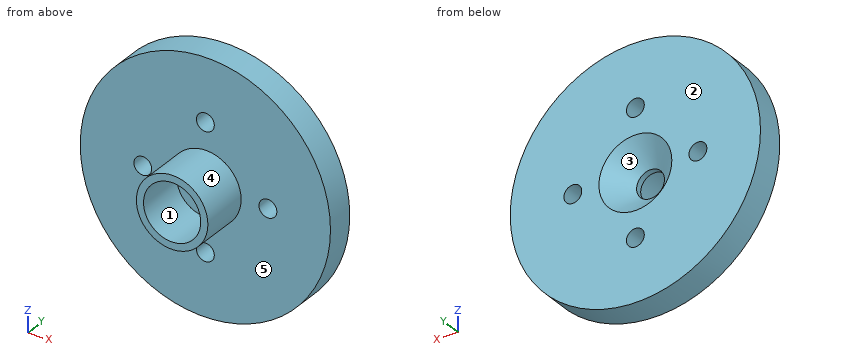
```python
from build123d import *

# Parameters (mm, degrees)
SKETCH1_R                                         = 17.5
BOSS_EXTRUDE1_DEPTH                               = 4
SKETCH2_R                                         = 5
SKETCH2_R_2                                       = 4
BOSS_EXTRUDE2_DEPTH                               = 6.9
SKETCH3_R                                         = 1.25
CUT_EXTRUDE1_DEPTH                                = 6.9
CSK_FOR_M3_5_FLAT_HEAD_MACHINE_SCREW1_D           = 3.9
CSK_FOR_M3_5_FLAT_HEAD_MACHINE_SCREW1_CSINK_D     = 10.2
CSK_FOR_M3_5_FLAT_HEAD_MACHINE_SCREW1_CSINK_ANGLE = 90
SKETCH6_R                                         = 1.25
CUT_EXTRUDE2_DEPTH                                = 6.9


with BuildPart() as part:
    # Sketch1 → Boss-Extrude1 (new body)
    with BuildSketch(Plane(origin=(0, 0, 0), x_dir=(1, 0, 0), z_dir=(0, 1, 0))):
        Circle(SKETCH1_R)
    extrude(amount=BOSS_EXTRUDE1_DEPTH)

    # Sketch2 → Boss-Extrude2 (add)
    with BuildSketch(Plane.XZ):
        Circle(SKETCH2_R)
        Circle(SKETCH2_R_2, mode=Mode.SUBTRACT)
    extrude(amount=BOSS_EXTRUDE2_DEPTH)

    # Sketch3 → Cut-Extrude1 (cut)
    with BuildSketch(Plane.XZ):
        with Locations((-8.75, 0)):
            Circle(SKETCH3_R)
        with Locations((8.75, 0)):
            Circle(SKETCH3_R)
    extrude(amount=-CUT_EXTRUDE1_DEPTH, mode=Mode.SUBTRACT)

    # CSK for M3.5 Flat Head Machine Screw1 (through all)
    with Locations(Plane(origin=(0, 4, 0), x_dir=(1, 0, 0), z_dir=(0, 1, 0))):
        with Locations((0, 0)):
            CounterSinkHole(CSK_FOR_M3_5_FLAT_HEAD_MACHINE_SCREW1_D / 2, CSK_FOR_M3_5_FLAT_HEAD_MACHINE_SCREW1_CSINK_D / 2, counter_sink_angle=CSK_FOR_M3_5_FLAT_HEAD_MACHINE_SCREW1_CSINK_ANGLE)

    # Sketch6 → Cut-Extrude2 (cut)
    with BuildSketch(Plane.XZ):
        with Locations((0, 8.75)):
            Circle(SKETCH6_R)
        with Locations((0, -8.75)):
            Circle(SKETCH6_R)
    extrude(amount=-CUT_EXTRUDE2_DEPTH, mode=Mode.SUBTRACT)


solid = part.part
```
CAD build for the part. Positions are in the model's coordinates, mm. Face numbers are marked on the shaded views. A direction names the side the tool comes from. Round coordinates to 2 decimals unless told otherwise and drop trailing zeros. Order: outer loops, then holes, each group sorted by start corner. A loop starts at its lowest first (then second) coordinate and runs counter-clockwise, first axis right, second up. Notation, with made-up numbers: (40, -31) - (48, -31) arc R6 cw to (48, -26) - close; hole circle Ø5 at (-40, 24.25). An arc over 180 degrees is marked (long way). Answer as CSV lines item,"result". Start each with the question number.
1. Pin check, flat tips, straight feed: pin 1 (10.5 mm diameter, centred on x = 0, z = 0, fed in from +Y); pin 2 (3 mm diameter, centred on x = -8.75, z = 0, fed in from -Y); pin 3 (6 mm diameter, centred on x = -4.5, y = 2.5, fed in from +Z); pin 4 (2 mm diameter, centred on x = 0, z = 8.75, fed in from -Y). Stop position of each tip, or through.
2. Saw through at C-C, the plane y = 2.25. Write the cut outline in (x, z).
3. Pull direction Z, two halves, no side cores. Call the marked faces 3, 4 and 5: +Z half, -Z half, draft (parallel to the pull), parting line (faces both ways), or undercut.
4. Drill centre lines: L1, parallel to Z at x = 0, y = -2.5; L2, parallel to Z at x = 0, y = 0.25; L3, parallel to Y at x = -5, z = 8.5. Where is each one in solid material? Low to high. Write a range as [from, to].
5. Saw through at D-D, the plane z = -8.75. Write the cut outline in (x, y), and give its area (3 significant figures).
6. Saw through at A-A, the plane x = 0. Write the cut outline in (y, z), and give its area (3 significant figures).
7. Tool access for the marked faces 1 and 2: list every direction of +Z, -Z, +X, -X, +Y, -Y with a clear straight run to the whole face (end or side of a thin tool).
8. Saw through at B-B, the plane z = 0. Write the cut outline in (x, y).
Model answer:
1,pin 1,"stops at y = 4"
1,pin 2,"stops at y = 0"
1,pin 3,"stops at z = 17.44"
1,pin 4,"passes through"
2,outline,"circle Ø35 at (0, 0); hole circle Ø2.5 at (-8.75, 0); hole circle Ø6.7 at (0, 0); hole circle Ø2.5 at (0, -8.75); hole circle Ø2.5 at (0, 8.75); hole circle Ø2.5 at (8.75, 0)"
3,face 3,"undercut"
3,face 4,"parting line"
3,face 5,"draft"
4,L1,"z = [-5, -4], [4, 5]"
4,L2,"z = [-17.5, -10], [-7.5, -1.95], [1.95, 7.5], [10, 17.5]"
4,L3,"y = [0, 4]"
5,outline,"(-15.16, 0) - (-1.25, 0) - (-1.25, 4) - (-15.16, 4) - close; (1.25, 0) - (15.16, 0) - (15.16, 4) - (1.25, 4) - close"
5,area,"111 mm²"
6,outline,"(-6.9, -5) - (0, -5) - (0, -7.5) - (4, -7.5) - (4, -5.1) - (0.85, -1.95) - (0, -1.95) - (0, -4) - (-6.9, -4) - close; (-6.9, 4) - (0, 4) - (0, 1.95) - (0.85, 1.95) - (4, 5.1) - (4, 7.5) - (0, 7.5) - (0, 5) - (-6.9, 5) - close; (0, -17.5) - (4, -17.5) - (4, -10) - (0, -10) - close; (0, 10) - (4, 10) - (4, 17.5) - (0, 17.5) - close"
6,area,"108 mm²"
7,face 1,"-Y"
7,face 2,"+Z, -Z, +X, -X, +Y"
8,outline,"(-17.5, 0) - (-10, 0) - (-10, 4) - (-17.5, 4) - close; (-7.5, 0) - (-5, 0) - (-5, -6.9) - (-4, -6.9) - (-4, 0) - (-1.95, 0) - (-1.95, 0.85) - (-5.1, 4) - (-7.5, 4) - close; (1.95, 0) - (4, 0) - (4, -6.9) - (5, -6.9) - (5, 0) - (7.5, 0) - (7.5, 4) - (5.1, 4) - (1.95, 0.85) - close; (10, 0) - (17.5, 0) - (17.5, 4) - (10, 4) - close"
